Input: part model. Units: mm. Frame: model coordinates. A direction names the side the tool comes from. Give positions to 0.01 mm unless a question says otherwise; leave off trailing zeros. Loops run counter-clockwise (first coordinate to the right, second up) from the corner with the lowest first, then second, coordinate; pieces in that order, holes last. Notation, with made-up numbers: M 18.5,-23 L 54.5,-23 A19 ccw 54.5,12 Z; hole C -8.75,22 d3. An arc over 180 degrees is marked long. Answer as a JSON object with one key per item and string values. Group by question number.
1) Section query B-B on y = 11. Return loops of the section in (x, z), plus the area to 3 significant figures.
2) Section query A-A on x = 48.5. Return loops of the section in (y, z), plus the area to 3 significant figures.
3) Ray query, L1, parallel to X at y = 14, z = 0; L2, parallel to Y at x = 41, z = 12.5; L3, parallel to X at y = 17.5, z = 10. Return the intervals inside material, ascending.
4) Draft query along Z for faces 5 (the cylindrical face through (28.3, -0.31, -26.01)), 6 (the flat face through (50, -18, 24)), 7 (the cylindrical face through (6.466, 9.675, -2.681)), 8 (the flat face through (26, 22, 2)). Return one class per face: +Z half, -Z half, draft (parallel to the pull), parting line (faces both ways), or undercut.
5) Section query D-D on x = -4. Return loops of the section in (y, z).
6) First-contact query: P1, Ø3, axis at x = 25.5, y = -3, coming from the +Z side; P2, Ø5, axis at y = -15, z = 8.5, coming from the -X side; P3, Ø23, axis at x = 2, z = -5.5, coming from the -Y side; P4, Ø21, axis at y = -8.5, z = 7.5, coming from the -X side. Flat tips, straight axial feed; report the tip coordinate or a pass-through.
7) Access query for faces 1 (the flat face through (51, -14, 17)), 2 (the flat face through (-3, 9, 18)), 3 (the flat face through (15, -13, 1)), 4 (the flat face through (64.217, -18.056, 21.138)). Directions: +Z, -Z, +X, -X, +Y, -Y. A direction counts if a zero-diameter tool reaches every point of the face in a straight line with its end or side. Return the directions, or none.
8) Section query C-C on z = -5.5. Return loops of the section in (x, y), plus the area to 3 significant figures.
from build123d import *

# Parameters (mm, degrees)
F0_R        = 7
F1_DEPTH    = 22
F3_DEPTH    = 69.1
F4_T4_DEPTH = 24
F2_W        = 40.4194121808
F2_H        = 21.5930561535
F5_DEPTH    = 72.2


# Not quite as in the source:
# - a fillet or chamfer that OpenCascade refuses, or shapes differently, is made with other operations: its cross-section is extruded or revolved along the edge and cut away or added


with BuildPart() as f1:
    # F0 (on Front) → F1 (new body, symmetric)
    with BuildSketch(Plane.XZ):
        with BuildLine():
            Line((-7, 18), (-14, 11))
            Line((-14, 11), (-14, -7))
            Line((-14, -7), (-7, -14))
            Line((-7, -14), (21.0666262554, -14))
            ThreePointArc((21.0666262554, -14), (24.3318620364, -15.2134137678), (26.0122649968, -18.2647058824))
            ThreePointArc((26.0122649968, -18.2647058824), (28.3490951999, -26.115672061), (32.7880673968, -33))
            Line((32.7880673968, -33), (38, -33))
            Line((38, -33), (67, 0))
            Line((67, 0), (67, 18.3546076061))
            Line((67, 18.3546076061), (61.3546076061, 24))
            Line((61.3546076061, 24), (38, 24))
            ThreePointArc((38, 24), (29.5749729609, 16.2760691513), (18.2430849879, 14.7832519053))
            Line((18.2430849879, 14.7832519053), (0, 18))
            Line((0, 18), (-7, 18))
        make_face()
        Circle(F0_R, mode=Mode.SUBTRACT)
        with Locations((53, 10)):
            Circle(F0_R, mode=Mode.SUBTRACT)
    extrude(amount=F1_DEPTH, both=True)

    # F2 (on Top) → F3 (cut)
    with BuildSketch(Plane.XY):
        Polygon((90.3841100792, -14), (90.3841100792, 10), (25.3584354958, 10), (25.3584354958, -14), (86.1629769206, -14), align=None)
    extrude(amount=F3_DEPTH, mode=Mode.SUBTRACT)

    # F4: fillet of radius 65.7 on 1 edges, made by hand


with BuildPart() as f4_tool2:
    # F4_s3 → F4_t4 (new body)
    with BuildSketch(Plane.XZ.offset(-10)):
        with BuildLine():
            ThreePointArc((67, 0), (44.8895413168, 3.8321555148), (25.3584354958, 14.88175752))
            Line((25.3584354958, 14.88175752), (24.5256098882, 13.8653926704))
            ThreePointArc((24.5256098882, 13.8653926704), (24.0444354958, 7.44087876), (24.0444354958, 0))
            Line((24.0444354958, 0), (25.3584354958, -1.314))
            Line((25.3584354958, -1.314), (67.0000056826, -1.314))
            Line((67.0000056826, -1.314), (67, 0))
        make_face()
    extrude(amount=F4_T4_DEPTH)

    split(bisect_by=Plane(origin=(37.8046632124, 0, -33.2222797927), x_dir=(0, 1, 0), z_dir=(-0.7511648984, 0, 0.6601146077)), keep=Keep.TOP)


with BuildPart() as f1_1:
    add(f1.part)

    # F4_t1: union F4_tool2
    add(f4_tool2.part)

    # F2 (on Top) → F5 (cut, symmetric)
    with BuildSketch(Plane.XY):
        with Locations((-5.2097060904, -13.7965280768)):
            Rectangle(F2_W, F2_H)
    extrude(amount=F5_DEPTH, both=True, mode=Mode.SUBTRACT)


solid = f1_1.part
Output:
{
 "1": {"outline": "M -14,-7 L -7,-14 L 21.07,-14 A5 cw 26.01,-18.26 A29 ccw 32.79,-33 L 38,-33 L 67,0 L 67,18.35 L 61.35,24 L 38,24 A19 cw 18.24,14.78 L 0,18 L -7,18 L -14,11 Z; hole C 0,0 d14; hole C 53,10 d14", "area": "2,610 mm^2"},
 "2": {"outline": "M -22,-21.05 L 22,-21.05 L 22,4.64 L 10,4.64 L 10,2.66 L -14,2.66 L -14,4.64 L -22,4.64 Z; M -22,15.36 L -14,15.36 L -14,24 L -22,24 Z; M 10,15.36 L 22,15.36 L 22,24 L 10,24 Z", "area": "1,260 mm^2"},
 "3": {"L1": "x = -14 to -7, 7 to 67", "L2": "y = -22 to -14, 10 to 22", "L3": "x = -14 to 46, 60 to 67"},
 "4": {"face 5": "-Z half", "face 6": "+Z half", "face 7": "undercut", "face 8": "draft"},
 "5": {"outline": "M -3,-14 L 22,-14 L 22,-5.74 L -3,-5.74 Z; M -3,5.74 L 22,5.74 L 22,18 L -3,18 Z"},
 "6": {"P1": "stops at z = 14.88", "P2": "stops at x = 15", "P3": "stops at y = -3", "P4": "stops at x = -14"},
 "7": {"face 1": "+Z, +X", "face 2": "+Z, -X, +Y, -Y", "face 3": "+Z, -Z, -X, -Y", "face 4": "+Z, +X, +Y, -Y"},
 "8": {"outline": "M -14,-3 L -4.33,-3 L -4.33,22 L -14,22 Z; M 4.33,-3 L 15,-3 L 15,-22 L 62.17,-22 L 62.17,22 L 4.33,22 Z", "area": "2,580 mm^2"}
}
